Could you check a few things on this model? Use its own coordinates, in mm. Face numbers are marked on the shaded views. A direction names the side the tool comes from. Round coordinates to 2 decimals unless told otherwise and drop trailing zeros. Order: outer loops, then holes, each group sorted by start corner. A loop starts at its lowest first (then second) coordinate and runs counter-clockwise, first axis right, second up. Notation, with made-up numbers: (53.25, 43.25) - (105.25, 43.25) arc R15 ccw to (105.25, 61.25) - close; hole circle Ø8 at (37.25, 68). An arc over 180 degrees is marked (long way). Return JSON: item names as keys, results as strings. Group by question number.
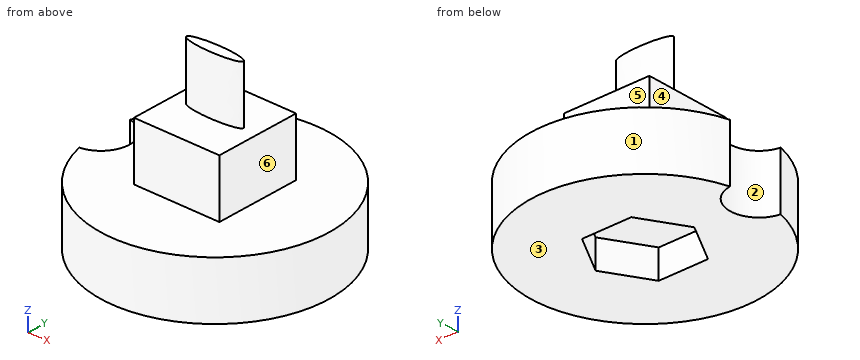
from build123d import *

# Parameters (mm, degrees)
F1_DEPTH = 25.4
F3_DEPTH = 25.4
F5_DEPTH = 25.4
F7_DEPTH = 12.7


with BuildPart() as f1:
    # F0 (on Top) → F1 (new body)
    with BuildSketch(Plane.XY):
        with BuildLine():
            ThreePointArc((-49.2125, 12.600391), (-38.1, 0), (-49.2125, -12.600391))
            ThreePointArc((-49.2125, -12.600391), (50.8, 0), (-49.2125, 12.600391))
        make_face()
    extrude(amount=F1_DEPTH)

    # F2 (on face) → F3 (join)
    with BuildSketch(Plane.XY.offset(25.4)):
        Polygon((0, 0), (-19.05, 19.05), (-19.05, -19.05), align=None)
        Polygon((19.05, 19.05), (-19.05, 19.05), (0, 0), align=None)
        Polygon((19.05, -19.05), (19.05, 19.05), (0, 0), align=None)
        Polygon((0, 0), (-19.05, -19.05), (19.05, -19.05), align=None)
    extrude(amount=F3_DEPTH)

    # F4 (on face) → F5 (join)
    with BuildSketch(Plane.XY.offset(50.8)):
        with BuildLine():
            add(Edge.make_bspline(
                [(-12.7, 0), (-12.7, -4.399409), (6.35, -2.199705), (25.4, 0), (6.35, 2.199705), (-12.7, 4.399409), (-12.7, 0)],
                knots=[0, 0, 0, 2.094395, 2.094395, 4.18879, 4.18879, 6.283185, 6.283185, 6.283185], degree=2, weights=[1, 0.5, 1, 0.5, 1, 0.5, 1]))
        make_face()
    extrude(amount=F5_DEPTH)

    # F6 (on Top) → F7 (cut)
    with BuildSketch(Plane.XY):
        with BuildLine():
            ThreePointArc((16.497784, -9.525), (18.400887, -4.930503), (19.05, 0))
            ThreePointArc((19.05, 0), (18.400887, 4.930503), (16.497784, 9.525))
            ThreePointArc((16.497784, 9.525), (9.525, 16.497784), (0, 19.05))
            ThreePointArc((0, 19.05), (-9.525, 16.497784), (-16.497784, 9.525))
            ThreePointArc((-16.497784, 9.525), (-19.05, 0), (-16.497784, -9.525))
            ThreePointArc((-16.497784, -9.525), (-9.525, -16.497784), (0, -19.05))
            ThreePointArc((0, -19.05), (9.525, -16.497784), (16.497784, -9.525))
        make_face()
        with BuildLine():
            ThreePointArc((16.497784, 9.525), (18.400887, 4.930503), (19.05, 0))
            ThreePointArc((19.05, 0), (18.400887, -4.930503), (16.497784, -9.525))
            Line((16.497784, -9.525), (21.997045, 0))
            Line((21.997045, 0), (16.497784, 9.525))
        make_face()
        with BuildLine():
            ThreePointArc((0, 19.05), (9.525, 16.497784), (16.497784, 9.525))
            Line((16.497784, 9.525), (10.998523, 19.05))
            Line((10.998523, 19.05), (0, 19.05))
        make_face()
        with BuildLine():
            Line((10.998523, -19.05), (16.497784, -9.525))
            ThreePointArc((16.497784, -9.525), (9.525, -16.497784), (0, -19.05))
            Line((0, -19.05), (10.998523, -19.05))
        make_face()
        with BuildLine():
            ThreePointArc((-16.497784, 9.525), (-9.525, 16.497784), (0, 19.05))
            Line((0, 19.05), (-10.998523, 19.05))
            Line((-10.998523, 19.05), (-16.497784, 9.525))
        make_face()
        with BuildLine():
            Line((-10.998523, -19.05), (0, -19.05))
            ThreePointArc((0, -19.05), (-9.525, -16.497784), (-16.497784, -9.525))
            Line((-16.497784, -9.525), (-10.998523, -19.05))
        make_face()
        with BuildLine():
            ThreePointArc((-16.497784, -9.525), (-19.05, 0), (-16.497784, 9.525))
            Line((-16.497784, 9.525), (-21.997045, 0))
            Line((-21.997045, 0), (-16.497784, -9.525))
        make_face()
    extrude(amount=F7_DEPTH, mode=Mode.SUBTRACT)


solid = f1.part
1) For the marked faces 4, 5 and 6, which set-ups out of +Z, -Z, +X, -X, +Y, -Y let a thin tool reach every point of the face, with its end or its side?
2) I want a section at B-B, the plane z = 36.5. List the corners of the cut face in (x, y) for me, plus the area to 3 significant figures.
3) I want a section at A-A, the plane y = -15. List the corners of the cut face in (x, z) for me.
4) I want a section at D-D, the plane y = 15.5. List the corners of the cut face in (x, z) for me.
5) I want a section at C-C, the plane x = -28. List the corners of the cut face in (y, z) for me, plus the area to 3 significant figures.
6) If I drill on line 1 along Z through (x, y) = (-42, 14.5); line 2 along Y through (x, z) = (-8, 37); line 3 along Y through (x, z) = (-42, 24.5), over which ranges is the centre line in solid material (lowest first)? Write a range as from..to.
7) We'd pull the mould along Y, two halves only. Please class the marked faces 1, 2 and 3: +Y half, -Y half, draft (parallel to the pull), parting line (faces both ways), or undercut.
8) Will these pins go through, and if not, where does the flat tip stop? pin 1 (8 mm diameter, centred on y = -16, z = 48, fed in from -X); pin 2 (3 mm diameter, centred on x = -17, y = 18, fed in from +Z); pin 3 (3 mm diameter, centred on y = 24, z = 20.5, fed in from +X); pin 4 (12 mm diameter, centred on x = 34, z = 35.5, fed in from -Y).
Outcome:
{
 "1": {"face 4": "+Z, -X, +Y, -Y", "face 5": "+Z, +X, -X, +Y", "face 6": "+Z, +X, +Y, -Y"},
 "2": {"outline": "(-19.05, -19.05) - (19.05, -19.05) - (19.05, 19.05) - (-19.05, 19.05) - close", "area": "1,450 mm^2"},
 "3": {"outline": "(-48.53, 0) - (-13.34, 0) - (-13.34, 12.7) - (13.34, 12.7) - (13.34, 0) - (48.53, 0) - (48.53, 25.4) - (19.05, 25.4) - (19.05, 50.8) - (-19.05, 50.8) - (-19.05, 25.4) - (-48.53, 25.4) - close"},
 "4": {"outline": "(-48.38, 0) - (-13.05, 0) - (-13.05, 12.7) - (13.05, 12.7) - (13.05, 0) - (48.38, 0) - (48.38, 25.4) - (19.05, 25.4) - (19.05, 50.8) - (-19.05, 50.8) - (-19.05, 25.4) - (-48.38, 25.4) - close"},
 "5": {"outline": "(-42.39, 0) - (42.39, 0) - (42.39, 25.4) - (-42.39, 25.4) - close", "area": "2,150 mm^2"},
 "6": {"line 1": "0..25.4", "line 2": "-19.05..19.05", "line 3": "-28.58..-9.16, 9.16..28.58"},
 "7": {"face 1": "parting line", "face 2": "undercut", "face 3": "draft"},
 "8": {"pin 1": "x = -19.05", "pin 2": "z = 50.8", "pin 3": "x = 45.55", "pin 4": "through"}
}
